Verification items for the finished model (mm, model axes). A direction names the side the tool comes from. Round coordinates to 2 decimals unless told otherwise and drop trailing zeros. Write each loop counter-clockwise with the first axis right and the second up, starting at its lowest first coordinate (ties: lowest second). Pieces come first, ordered by that corner, then holes. Notation, with made-up numbers: M -16,56.5 L 13,56.5 A22 cw 13,68.5 Z; hole C 87,1.25 d9. An arc over 180 degrees is marked long. One line per item, written item: value. Start each with the question number.
from build123d import *

# Parameters (mm, degrees)
F0_W     = 1219.2
F0_H     = 63.5
F1_DEPTH = 19.05
F0_H_2   = 25.4
F2_DEPTH = 19.05
F3_SIZE2 = 38.1
F3_SIZE  = 19.05


with BuildPart() as f1:
    # F0 (on Top) → F1 (new body)
    with BuildSketch(Plane.XY):
        with Locations((353.564252, 15.255763)):
            Rectangle(F0_W, F0_H)
    extrude(amount=F1_DEPTH)

    # F0 (on Top) → F2 (join)
    with BuildSketch(Plane.XY):
        with Locations((353.564252, 15.255763)):
            Rectangle(F0_W, F0_H)
        with Locations((353.564252, -29.194237)):
            Rectangle(F0_W, F0_H_2)
    extrude(amount=-F2_DEPTH)

    # F3
    f3_edges = [f1.edges().sort_by_distance(p)[0] for p in [
        (353.564252, 47.005763, 19.05),
    ]]
    chamfer(f3_edges, length=F3_SIZE, length2=F3_SIZE2)


solid = f1.part
1) Cross-section at C-C (z = 9.5). Record the boundary of the cut face in (x, y), then the cut area to 3 significant figures.
2) Cross-section at A-A (x = -146). Record the boundary of the cut face in (y, z), then the cut area to 3 significant figures.
3) Cross-section at B-B (y = -32). Record the boundary of the cut face in (x, z), then the cut area to 3 significant figures.
4) Gauge pin test, flat ends, axial feed: pin 1 Ø9.5 at (x, z) = (132.5, 11) entering from -Y; pin 2 Ø8 at (x, z) = (583.5, 8) entering from +Y; pin 3 Ø12.5 at (x, y) = (324.5, -24) entering from +Z. Record the tip position at first contact, or that the pin passes through.
5) Thickness scan on line 1 (Z direction, x = 458, y = -36); line 2 (Z direction, x = 259, y = 37); line 3 (Y direction, x = 824.5, z = 5). Record the ranges inside material, lowest first.
6) Access from +Z, -Z, +X, -X, +Y, -Y to the whole of each face (thin tool, end or side, straight path). Record for faces 1 (the flat face through (345, -4, 19.05)), 2 (the flat face through (345, -16.494, 9)).
Results below:
1. outline: M -256.04,-16.49 L 963.16,-16.49 L 963.16,28.01 L -256.04,28.01 Z
1. area: 54,300 mm²
2. outline: M -41.89,-19.05 L 47.01,-19.05 L 47.01,0 L 8.91,19.05 L -16.49,19.05 L -16.49,0 L -41.89,0 Z
2. area: 2,540 mm²
3. outline: M -256.04,-19.05 L 963.16,-19.05 L 963.16,0 L -256.04,0 Z
3. area: 23,200 mm²
4. pin 1: stops at y = -16.49
4. pin 2: stops at y = 39.01
4. pin 3: stops at z = 0
5. line 1: z = -19.05 to 0
5. line 2: z = -19.05 to 5
5. line 3: y = -16.49 to 37.01
6. face 1: +Z, +X, -X, +Y, -Y
6. face 2: +Z, +X, -X, -Y
